Read the model definition and answer for the solid it produces. Units are mm, in the model's axes. A direction names the side the tool comes from. Coordinates: 2 decimals unless noted, no trailing zeros. Order: outer loops, then holes, each group sorted by start corner. A loop starts at its lowest first (then second) coordinate and runs counter-clockwise, first axis right, second up.
Autodesk Fusion 360 part; units mm, degrees
sketch "Sketch1" plane through (0, 0, 0) normal (1, 0, 0) x (0, 0, -1)
  line L0 (0, 0) -> (-4, 0)
  line L1 (-4, 0) -> (-4, 30)
  line L2 (-4, 30) -> (0, 30)
  line L3 (0, 30) -> (0, 0)
  line L4 (-4, 30) -> (-8, 30)
  line L5 (-8, 30) -> (-8, 0)
  line L6 (-8, 0) -> (-4, 0)
  line L7 (-4, 0) -> (-4, 30)
  line L8 (-4, 30) -> (-6, 30)
  line L9 (-6, 30) -> (-6, 28)
  line L10 (-6, 28) -> (-4, 28)
  line L11 (-4, 28) -> (-4, 30)
  line L12 (-4, 0) -> (-8, 0)
  line L13 (-8, 0) -> (-8, 2)
  line L14 (-8, 2) -> (-4, 2)
  line L15 (-4, 2) -> (-4, 0)
  line L16 (-6, 28) -> (-8, 2)
  spline S0 degree 5 poles (-4, 2) (-4.0818, 2.52) (-4.2384, 3.56) (-4.4517, 5.12) (-4.6926, 7.2) (-4.9161, 9.8) (-5.0551, 12.4) (-5.1027, 15) (-5.0551, 17.6) (-4.9161, 20.2) (-4.6926, 22.8) (-4.4517, 24.88) (-4.2384, 26.44) (-4.0818, 27.48) (-4, 28) knots 0 0 0 0 0 0 0.1 0.2 0.3 0.4 0.5 0.6 0.7 0.8 0.9 1 1 1 1 1 1
  point P0 (-5.079, 15)
  dimension "d1" = 4
  dimension "d2" = 30
  dimension "d3" = 4
  dimension "d4" = 30
  dimension "d5" = 2
  dimension "d6" = 2
  dimension "d7" = 2
revolve "Revolve1" add sketch "Sketch1" angle 360 about axis through (0, 30, 0) along (0, -1, 0) contours L1 L5 L6 L7 L12 L13 L14 L15 | L10 L14 L16 S0 | L1 L4 L7 L8 L9 L10 L11
sketch "Sketch2" plane through (0, 0, 0) normal (0, -1, 0) x (1, 0, 0)
  circle A0 centre (0, 0) radius 4
  circle A1 centre (0, 0) radius 8
  line L0 (0, 0) -> (10, 0)
  line L1 (10, 0) -> (10, 10)
  line L2 (10, 10) -> (0, 10)
  line L3 (0, 10) -> (0, 0)
  line L4 (0, 0) -> (-10, 0)
  line L5 (-10, 0) -> (-10, 10)
  line L6 (-10, 10) -> (0, 10)
  line L7 (0, 10) -> (0, 0)
  line L8 (0, 0) -> (-10, 0)
  line L9 (-10, 0) -> (-10, -10)
  line L10 (-10, -10) -> (0, -10)
  line L11 (0, -10) -> (0, 0)
  line L12 (0, 0) -> (10, 0)
  line L13 (10, 0) -> (10, -10)
  line L14 (10, -10) -> (0, -10)
  line L15 (0, -10) -> (0, 0)
  line L16 (0, 15) -> (-15, 15)
  line L17 (-15, 15) -> (0, 15)
  line L18 (0, 15) -> (15, 15)
  line L19 (-17.5, 17.5) -> (17.5, 17.5)
  line L20 (17.5, 17.5) -> (17.5, 10)
  line L21 (17.5, 10) -> (-17.5, 10)
  line L22 (-17.5, 10) -> (-17.5, 17.5)
  circle A2 centre (-15, 15) radius 1
  circle A3 centre (15, 15) radius 1
  line L23 (-10, -8) -> (10, -8)
  circle A4 centre (0, 0) radius 10
  dimension "d9" = 15
  dimension "d10" = 15
  dimension "d11" = 2
  dimension "d12" = 2
extrude "Extrude1" add sketch "Sketch2" against normal blind 2 contours A1 L0 L12 L23 A4 | A1 L0 L3 L7 L12 A4 | A1 L3 L4 L7 L8 A4 | A1 L4 L8 L23 A4 | L11 L15 L23 A4 | L11 L15 L23 A4 | L1 L2 L21 A4 | L2 L6 L19 L20 L21 L22 | L5 L6 L21 A4
sketch "Sketch3" plane through (0, 0, 0) normal (1, 0, 0) x (0, 0, -1)
  line L0 (-6, 30) -> (-16, 2)
  line L1 (-16, 2) -> (-7, 2)
  line L2 (-7, 2) -> (-5, 28)
  line L3 (-5, 28) -> (-5, 30)
  line L4 (-5, 30) -> (-6, 30)
extrude "Extrude2" add sketch "Sketch3" along normal mid plane 2
sketch "Sketch4" plane through (0, 0, 0) normal (1, 0, 0) x (0, 0, -1)
  line L0 (6, 30) -> (10, 2)
  line L1 (10, 2) -> (7, 2)
  line L2 (7, 2) -> (5, 28)
  line L3 (5, 28) -> (5, 30)
  line L4 (5, 30) -> (6, 30)
extrude "Extrude3" add sketch "Sketch4" along normal mid plane 2
sketch "Sketch5" plane through (0, 0, 0) normal (0, -1, 0) x (1, 0, 0)
  arc A0 (-10, 0) -> (10, 0) centre (0, 0) ccw
  line L0 (10, 0) -> (10, 10)
  line L1 (10, 10) -> (17.5, 10)
  line L2 (17.5, 10) -> (17.5, 17.5)
  line L3 (17.5, 17.5) -> (-17.5, 17.5)
  line L4 (-17.5, 17.5) -> (-17.5, 10)
  line L5 (-17.5, 10) -> (-10, 10)
  line L6 (-10, 10) -> (-10, 0)
  circle A1 centre (15, 15) radius 1
  circle A2 centre (-15, 15) radius 1
  circle A3 centre (0, 0) radius 4
  line L7 (-17.5, 10) -> (-8.6154, -5.0769)
  line L8 (17.5, 10) -> (8.6154, -5.0769)
extrude "Extrude4" add sketch "Sketch5" against normal blind 2 contours A0 L5 L6 L7 | A0 L0 L1 L8
sketch "Sketch6" plane through (0, 0, 0) normal (0, -1, 0) x (1, 0, 0)
  arc A0 (-8.6154, -5.0769) -> (8.6154, -5.0769) centre (0, 0) ccw
  line L0 (8.6154, -5.0769) -> (17.5, 10)
  line L1 (17.5, 10) -> (17.5, 17.5)
  line L2 (17.5, 17.5) -> (-17.5, 17.5)
  line L3 (-17.5, 17.5) -> (-17.5, 10)
  line L4 (-17.5, 10) -> (-8.6154, -5.0769)
  circle A1 centre (15, 15) radius 1
  circle A2 centre (-15, 15) radius 1
  circle A3 centre (0, 0) radius 4
  line L5 (10, -1) -> (15, -1)
  line L6 (15, -1) -> (15, 1)
  line L7 (15, 1) -> (10, 1)
  line L8 (10, 1) -> (10, -1)
  line L9 (-10, -1) -> (-15, -1)
  line L10 (-15, -1) -> (-15, 1)
  line L11 (-15, 1) -> (-10, 1)
  line L12 (-10, 1) -> (-10, -1)
extrude "Extrude5" add sketch "Sketch6" against normal blind 2 contours L4 L9 L10 L11 | L0 L5 L6 L7
sketch "Sketch7" plane through (0, 2, 0) normal (0, 1, 0) x (-1, 0, 0)
  line L0 (1, -7.9373) -> (1, -9.9499)
  arc A0 (1, -9.9499) -> (8.6154, -5.0769) centre (0, 0) ccw
  line L1 (8.6154, -5.0769) -> (11.0179, -1)
  line L2 (11.0179, -1) -> (15, -1)
  line L3 (15, -1) -> (15, 1)
  line L4 (15, 1) -> (12.1964, 1)
  line L5 (12.1964, 1) -> (17.5, 10)
  line L6 (17.5, 10) -> (17.5, 17.5)
  line L7 (17.5, 17.5) -> (-17.5, 17.5)
  line L8 (-17.5, 17.5) -> (-17.5, 10)
  line L9 (-17.5, 10) -> (-12.1964, 1)
  line L10 (-12.1964, 1) -> (-15, 1)
  line L11 (-15, 1) -> (-15, -1)
  line L12 (-15, -1) -> (-11.0179, -1)
  line L13 (-11.0179, -1) -> (-8.6154, -5.0769)
  arc A1 (-8.6154, -5.0769) -> (-1, -9.9499) centre (0, 0) ccw
  line L14 (-1, -9.9499) -> (-1, -7.9373)
  arc A2 (-1, 7.9373) -> (-1, -7.9373) centre (0, 0) ccw
  line L15 (-1, 7.9373) -> (-1, 16)
  line L16 (-1, 16) -> (1, 16)
  line L17 (1, 16) -> (1, 7.9373)
  arc A3 (1, -7.9373) -> (1, 7.9373) centre (0, 0) ccw
  circle A4 centre (15, 15) radius 1
  circle A5 centre (-15, 15) radius 1
  line L18 (15, -1) -> (13.5, -1)
  line L19 (13.5, -1) -> (13.5, 1)
  line L20 (13.5, 1) -> (15, 1)
  line L21 (15, 1) -> (15, -1)
  line L22 (-15, -1) -> (-13.5, -1)
  line L23 (-13.5, -1) -> (-13.5, 1)
  line L24 (-13.5, 1) -> (-15, 1)
  line L25 (-15, 1) -> (-15, -1)
  dimension "d23" = 1.5
  dimension "d24" = 1.5
extrude "Extrude6" add sketch "Sketch7" along normal blind 2 contours L2 L3 L4 L18 L19 L20 L21 | L10 L11 L12 L22 L23 L24 L25
sketch "Sketch8" plane through (0, 0, 0) normal (0, -1, 0) x (1, 0, 0)
  arc A0 (-8.6154, -5.0769) -> (8.6154, -5.0769) centre (0, 0) ccw
  line L0 (8.6154, -5.0769) -> (11.0179, -1)
  line L1 (11.0179, -1) -> (15, -1)
  line L2 (15, -1) -> (15, 1)
  line L3 (15, 1) -> (12.1964, 1)
  line L4 (12.1964, 1) -> (17.5, 10)
  line L5 (17.5, 10) -> (17.5, 17.5)
  line L6 (17.5, 17.5) -> (-17.5, 17.5)
  line L7 (-17.5, 17.5) -> (-17.5, 10)
  line L8 (-17.5, 10) -> (-12.1964, 1)
  line L9 (-12.1964, 1) -> (-15, 1)
  line L10 (-15, 1) -> (-15, -1)
  line L11 (-15, -1) -> (-11.0179, -1)
  line L12 (-11.0179, -1) -> (-8.6154, -5.0769)
  circle A1 centre (15, 15) radius 1
  circle A2 centre (-15, 15) radius 1
  circle A3 centre (0, 0) radius 4
  line L13 (-17.5, 15.0174) -> (17.5, 15.0174)
  line L14 (17.5, 15.0174) -> (17.5, 30.0174)
  line L15 (17.5, 30.0174) -> (-17.5, 30.0174)
  line L16 (-17.5, 30.0174) -> (-17.5, 15.0174)
  dimension "d27" = 35
  dimension "d28" = 15
extrude "Extrude7" add sketch "Sketch8" against normal blind 2 contours L6 L14 L15 L16
sketch "Sketch9" plane through (0, 2, 0) normal (0, 1, 0) x (-1, 0, 0)
  circle A0 centre (-15, 15) radius 1
  circle A1 centre (15, 15) radius 1
  line L0 (13.5, -1) -> (13.5, 1)
  line L1 (13.5, 1) -> (12.1964, 1)
  line L2 (12.1964, 1) -> (17.5, 10)
  line L3 (17.5, 10) -> (17.5, 30.0174)
  line L4 (17.5, 30.0174) -> (-17.5, 30.0174)
  line L5 (-17.5, 30.0174) -> (-17.5, 10)
  line L6 (-17.5, 10) -> (-12.1964, 1)
  line L7 (-12.1964, 1) -> (-13.5, 1)
  line L8 (-13.5, 1) -> (-13.5, -1)
  line L9 (-13.5, -1) -> (-11.0179, -1)
  line L10 (-11.0179, -1) -> (-8.6154, -5.0769)
  arc A2 (-8.6154, -5.0769) -> (-1, -9.9499) centre (0, 0) ccw
  line L11 (-1, -9.9499) -> (-1, -7.9373)
  arc A3 (-1, 7.9373) -> (-1, -7.9373) centre (0, 0) ccw
  line L12 (-1, 7.9373) -> (-1, 16)
  line L13 (-1, 16) -> (1, 16)
  line L14 (1, 16) -> (1, 7.9373)
  arc A4 (1, -7.9373) -> (1, 7.9373) centre (0, 0) ccw
  line L15 (1, -7.9373) -> (1, -9.9499)
  arc A5 (1, -9.9499) -> (8.6154, -5.0769) centre (0, 0) ccw
  line L16 (8.6154, -5.0769) -> (11.0179, -1)
  line L17 (11.0179, -1) -> (13.5, -1)
  line L18 (15, 25) -> (10, 25)
  line L19 (10, 25) -> (10, 30)
  line L20 (10, 30) -> (15, 30)
  line L21 (15, 30) -> (15, 25)
  line L22 (-15, 25) -> (-10, 25)
  line L23 (-10, 25) -> (-10, 30)
  line L24 (-10, 30) -> (-15, 30)
  line L25 (-15, 30) -> (-15, 25)
  line L26 (-10, 25) -> (-1, 7.9373)
  line L27 (-15, 25) -> (-5.0752, 6.184)
  line L28 (10, 25) -> (1, 7.9373)
  line L29 (15, 25) -> (5.0752, 6.184)
  dimension "d31" = 5
  dimension "d32" = 5
extrude "Extrude8" add sketch "Sketch9" along normal blind 15 contours L18 L19 L20 L21 | L22 L23 L24 L25
sketch "Sketch10" plane through (15, 0, 0) normal (1, 0, 0) x (0, 0, -1)
  line L0 (-30, 2) -> (-25, 2)
  line L1 (-25, 2) -> (-25, 17)
  line L2 (-25, 17) -> (-30, 17)
  line L3 (-30, 17) -> (-30, 2)
  line L4 (-25, 17) -> (-20, 17)
  line L5 (-20, 17) -> (-20, 2)
  line L6 (-20, 2) -> (-25, 2)
  line L7 (-25, 2) -> (-25, 17)
  line L8 (-25, 17) -> (-20, 2)
extrude "Extrude9" add sketch "Sketch10" against normal blind 5 contours L1 L6 L7 L8
sketch "Sketch11" plane through (-15, 0, 0) normal (-1, 0, 0) x (0, 0, 1)
  line L0 (25, 2) -> (30, 2)
  line L1 (30, 2) -> (30, 17)
  line L2 (30, 17) -> (25, 17)
  line L3 (25, 17) -> (25, 2)
  line L4 (25, 17) -> (20, 17)
  line L5 (20, 17) -> (20, 2)
  line L6 (20, 2) -> (25, 2)
  line L7 (25, 2) -> (25, 17)
  line L8 (25, 17) -> (20, 2)
extrude "Extrude10" add sketch "Sketch11" against normal blind 5 contours L3 L6 L7 L8
1) Which of the six approach directions +Z, -Z, +X, -X, +Y, -Y give full straight-line access (tool end or side, diameter ignored) to faces 4 (the flat face through (15, 10, 26)), 5 (the flat face through (-10, 10, 26)), 6 (the flat face through (13.5, 3, 0))?
A:
face 4: +Z, -Z, +X, +Y
face 5: +Z, -Z, +Y
face 6: -Z, +Y
2) A cutting plane is placed at A-A, the plane z = 15. Determine the outline of the cut face in (x, y).
A:
outline: (-17.5, 0) - (-16, 0) - (-16, 2) - (-17.5, 2) - close; (-14, 0) - (14, 0) - (14, 2) - (1, 2) - (1, 4.8) - (-1, 4.8) - (-1, 2) - (-14, 2) - close; (16, 0) - (17.5, 0) - (17.5, 2) - (16, 2) - close
3) Flat-ended cylindrical pins translate along their axes: pin 1 Ø6 at (y, z) = (20, -4.5) entering from -X; pin 2 Ø0.6 at (y, z) = (3, -0.5) entering from +X; pin 3 Ø0.8 at (x, y) = (-14, 2.5) entering from +Z. Find the tip coordinate at first contact, or state that the pin passes through.
A:
pin 1: stops at x = -6.48
pin 2: stops at x = 15
pin 3: stops at z = 30
4) A cutting plane is placed at C-C, the plane z = 26. Determine the outline of the cut face in (x, y), and give its area (3 significant figures).
A:
outline: (-17.5, 0) - (17.5, 0) - (17.5, 2) - (15, 2) - (15, 17) - (10, 17) - (10, 2) - (-10, 2) - (-10, 17) - (-15, 17) - (-15, 2) - (-17.5, 2) - close
area: 220 mm2
5) Determine the mould class of faces 1 (the flat face through (-4, 2, 15)), 2 (the flat face through (0, 16, 11)), 3 (the flat face through (14.885, 0.986, 5.563)) for opening direction X: pulls with the +X half, pulls with the -X half, needs draft (parallel to the pull), parting line crosses it, or undercut.
A:
face 1: undercut
face 2: needs draft
face 3: pulls with the +X half
6) Straight lines are drawn through the part: line 1 (Z direction, x = 0, y = 0.55); line 2 (X direction, y = 1.1, z = 0); line 3 (X direction, y = 11.5, z = 23.5). For each, find the intervals that lie inside material, in ascending order.
A:
line 1: z = -10 to -4, 4 to 30.02
line 2: x = -15 to -4, 4 to 15
line 3: x = -15 to -10, 10 to 15
7) A cutting plane is placed at B-B, the plane y = 6.5. State how many separate pieces and enclosed holes the cut face has, and give its area (3 significant figures).
A:
separate pieces: 3
enclosed holes: 1
area: 220 mm2
